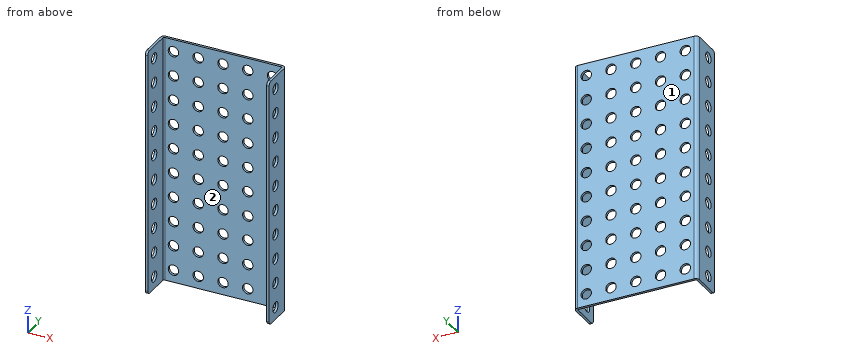
from build123d import *

# Parameters (mm, degrees)
PAD_DEPTH       = 100
FILLET_R        = 1.5
FILLET001_R     = 1.5
FILLET002_R     = 1.5
FILLET003_R     = 1.5
SKETCH001_R     = 2.1
POCKET_DEPTH    = 50.001
SKETCH002_R     = 2.1
POCKET001_DEPTH = 13.401


with BuildPart() as part:
    # Sketch → Pad (new body)
    with BuildSketch(Plane.XY):
        with BuildLine():
            Line((0, 0), (0, 11.9))
            ThreePointArc((1.5, 13.4), (0.43934, 12.96066), (0, 11.9))
            Line((1.5, 13.4), (48.5, 13.4))
            ThreePointArc((50, 11.9), (49.56066, 12.96066), (48.5, 13.4))
            Line((50, 11.9), (50, 0))
            Line((49, 0), (50, 0))
            Line((49, 11.9), (49, 0))
            ThreePointArc((49, 11.9), (48.853553, 12.253553), (48.5, 12.4))
            Line((1.5, 12.4), (48.5, 12.4))
            ThreePointArc((1.5, 12.4), (1.146447, 12.253553), (1, 11.9))
            Line((1, 0), (1, 11.9))
            Line((0, 0), (1, 0))
        make_face()
    extrude(amount=PAD_DEPTH)

    # Fillet
    fillet_edges = [part.edges().sort_by_distance(p)[0] for p in [
        (49.5, 0, 0),
    ]]
    fillet(fillet_edges, radius=FILLET_R)

    # Fillet001
    fillet001_edges = [part.edges().sort_by_distance(p)[0] for p in [
        (0.5, 0, 0),
    ]]
    fillet(fillet001_edges, radius=FILLET001_R)

    # Fillet002
    fillet002_edges = [part.edges().sort_by_distance(p)[0] for p in [
        (49.5, 0, 100),
    ]]
    fillet(fillet002_edges, radius=FILLET002_R)

    # Fillet003
    fillet003_edges = [part.edges().sort_by_distance(p)[0] for p in [
        (0.5, 0, 100),
    ]]
    fillet(fillet003_edges, radius=FILLET003_R)

    # Sketch001 → Pocket (cut, through all)
    with BuildSketch(Plane(origin=(0, 0, 0), x_dir=(0, -1, 0), z_dir=(-1, 0, 0))):
        with Locations((-5, 5)):
            Circle(SKETCH001_R)
        with Locations((-5, 15)):
            Circle(SKETCH001_R)
        with Locations((-5, 25)):
            Circle(SKETCH001_R)
        with Locations((-5, 35)):
            Circle(SKETCH001_R)
        with Locations((-5, 45)):
            Circle(SKETCH001_R)
        with Locations((-5, 55)):
            Circle(SKETCH001_R)
        with Locations((-5, 65)):
            Circle(SKETCH001_R)
        with Locations((-5, 75)):
            Circle(SKETCH001_R)
        with Locations((-5, 85)):
            Circle(SKETCH001_R)
        with Locations((-5, 95)):
            Circle(SKETCH001_R)
    extrude(amount=-POCKET_DEPTH, mode=Mode.SUBTRACT)

    # Sketch002 → Pocket001 (cut, through all)
    with BuildSketch(Plane(origin=(0, 13.4, 0), x_dir=(-1, 0, 0), z_dir=(0, 1, 0))):
        with Locations((-5, 5)):
            Circle(SKETCH002_R)
        with Locations((-15, 5)):
            Circle(SKETCH002_R)
        with Locations((-25, 5)):
            Circle(SKETCH002_R)
        with Locations((-35, 5)):
            Circle(SKETCH002_R)
        with Locations((-45, 5)):
            Circle(SKETCH002_R)
        with Locations((-45, 15)):
            Circle(SKETCH002_R)
        with Locations((-45, 25)):
            Circle(SKETCH002_R)
        with Locations((-45, 35)):
            Circle(SKETCH002_R)
        with Locations((-45, 45)):
            Circle(SKETCH002_R)
        with Locations((-45, 55)):
            Circle(SKETCH002_R)
        with Locations((-45, 65)):
            Circle(SKETCH002_R)
        with Locations((-45, 75)):
            Circle(SKETCH002_R)
        with Locations((-45, 85)):
            Circle(SKETCH002_R)
        with Locations((-45, 95)):
            Circle(SKETCH002_R)
        with Locations((-35, 15)):
            Circle(SKETCH002_R)
        with Locations((-35, 25)):
            Circle(SKETCH002_R)
        with Locations((-35, 35)):
            Circle(SKETCH002_R)
        with Locations((-35, 45)):
            Circle(SKETCH002_R)
        with Locations((-35, 55)):
            Circle(SKETCH002_R)
        with Locations((-35, 65)):
            Circle(SKETCH002_R)
        with Locations((-35, 75)):
            Circle(SKETCH002_R)
        with Locations((-35, 85)):
            Circle(SKETCH002_R)
        with Locations((-35, 95)):
            Circle(SKETCH002_R)
        with Locations((-25, 15)):
            Circle(SKETCH002_R)
        with Locations((-25, 25)):
            Circle(SKETCH002_R)
        with Locations((-25, 35)):
            Circle(SKETCH002_R)
        with Locations((-25, 45)):
            Circle(SKETCH002_R)
        with Locations((-25, 55)):
            Circle(SKETCH002_R)
        with Locations((-25, 65)):
            Circle(SKETCH002_R)
        with Locations((-25, 75)):
            Circle(SKETCH002_R)
        with Locations((-25, 85)):
            Circle(SKETCH002_R)
        with Locations((-25, 95)):
            Circle(SKETCH002_R)
        with Locations((-15, 15)):
            Circle(SKETCH002_R)
        with Locations((-15, 25)):
            Circle(SKETCH002_R)
        with Locations((-15, 35)):
            Circle(SKETCH002_R)
        with Locations((-15, 45)):
            Circle(SKETCH002_R)
        with Locations((-15, 55)):
            Circle(SKETCH002_R)
        with Locations((-15, 65)):
            Circle(SKETCH002_R)
        with Locations((-15, 75)):
            Circle(SKETCH002_R)
        with Locations((-15, 85)):
            Circle(SKETCH002_R)
        with Locations((-15, 95)):
            Circle(SKETCH002_R)
        with Locations((-5, 15)):
            Circle(SKETCH002_R)
        with Locations((-5, 25)):
            Circle(SKETCH002_R)
        with Locations((-5, 35)):
            Circle(SKETCH002_R)
        with Locations((-5, 45)):
            Circle(SKETCH002_R)
        with Locations((-5, 55)):
            Circle(SKETCH002_R)
        with Locations((-5, 65)):
            Circle(SKETCH002_R)
        with Locations((-5, 75)):
            Circle(SKETCH002_R)
        with Locations((-5, 85)):
            Circle(SKETCH002_R)
        with Locations((-5, 95)):
            Circle(SKETCH002_R)
    extrude(amount=-POCKET001_DEPTH, mode=Mode.SUBTRACT)


solid = part.part
Source: CAD feature listing. Evaluate the final solid. Frame: model axes, mm. Face numbers are marked on the shaded views. Give positions to 0.01 mm unless a question says otherwise; leave off trailing zeros. Write each loop counter-clockwise with the first axis right and the second up, starting at its lowest first coordinate (ties: lowest second). Pieces come first, ordered by that corner, then holes. Notation, with made-up numbers: M -13,-38 L 31,-38 A30 ccw 31,-5 Z; hole C 72.25,88 d8. An arc over 180 degrees is marked long. Return JSON: item names as keys, results as strings. Group by question number.
1) Cut plane A-A, the plane y = 9.5. Output: boundary loops of the cut face in (x, z).
2) Pull-direction query (X, two-part tool) for the marked faces 1 and 2; classes: pulls with the +X half, pulls with the -X half, needs draft (parallel to the pull), parting line crosses it, or undercut.
3) Pin query (flat end, axial travel): P1, Ø4, axis at x = 45, z = 65, coming from the -Y side; P2, Ø5, axis at x = 5, z = 5, coming from the -Y side. Return the tip coordinate at first contact, or that it passes through.
4) Material intervals for line 1 along X through (y, z) = (6.25, 49.5); line 2 along Y through (x, z) = (16, 23), sorted ascending. Write a range as [from, to].
5) Cut plane B-B, the plane x = 45. Give the number of separate pieces and of enclosed holes in the cut face, plus the area to 3 significant figures.
6) Cut plane D-D, the plane z = 91. Output: boundary loops of the cut face in (x, y), plus the area to 3 significant figures.
Recorded:
{
 "1": {"outline": "M 0,0 L 1,0 L 1,100 L 0,100 Z; M 49,0 L 50,0 L 50,100 L 49,100 Z"},
 "2": {"face 1": "needs draft", "face 2": "undercut"},
 "3": {"P1": "passes through", "P2": "stops at y = 12.4"},
 "4": {"line 1": "x = [0, 1], [49, 50]", "line 2": "y = [12.4, 13.4]"},
 "5": {"separate pieces": "11", "enclosed holes": "0", "area": "58.0 mm²"},
 "6": {"outline": "M 0,0 L 1,0 L 1,11.9 A0.5 cw 1.5,12.4 L 48.5,12.4 A0.5 cw 49,11.9 L 49,0 L 50,0 L 50,11.9 A1.5 ccw 48.5,13.4 L 1.5,13.4 A1.5 ccw 0,11.9 Z", "area": "73.9 mm²"}
}
